Verification items for this drawing (mm, ordinates from the low corner). A direction names the side the tool comes from. Round coordinates to 2 decimals unless told otherwise and drop trailing zeros. Order: outer loops, then holes, each group sorted by start corner. A loop starts at its lowest first (then second) coordinate and runs counter-clockwise, first axis right, second up. Notation, with made-up numbers: (-20, -30) -> (6, -30) arc R8 cw to (6, -23) -> close; hole circle Ø3 at (-25.5, -0.75). An arc over 180 degrees is marked (long way). Use a Markdown table: item, result. Add a question column.
Item 1: Gauge pin test, flat ends, axial feed: pin 1 Ø3 at (x, y) = (14, 5.5) entering from -Z; pin 2 Ø3 at (x, z) = (11, 10) entering from +Y; pin 3 Ø2 at (y, z) = (3.5, 14) entering from -X. Record the tip position at first contact, or that the pin passes through.
Item 2: Sectioned sample at D-D, the plane y = 5.75. Record the cut outline in (x, z).
Item 3: Sectioned sample at C-C, the plane y = 0.5. Record the cut outline in (x, z), and give its area (3 significant figures).
Item 4: Set-up check for the marked faces 1 and 2: record each of +Z, -Z, +X, -X, +Y, -Y from which the full face is reachable in a straight line by a thin tool's end or side.
Item 5: Mould release check, pull along X, two halves, no side actions. Record for the marked faces 3, 4 and 5: pulls with the +X half, pulls with the -X half, needs draft (parallel to the pull), parting line crosses it, or undercut.
Item 6: Sectioned sample at A-A, the plane x = 10. Record the cut outline in (y, z), and give its area (3 significant figures).
Item 7: Material ranges on probe 1 along Z at (x, y) = (10, 5.1); probe 2 along Y at (x, z) = (3.5, 13.5), recorded low to high. Write a range as [from, to].
Item 8: Sectioned sample at B-B, the plane z = 10. Record the cut outline in (x, y).
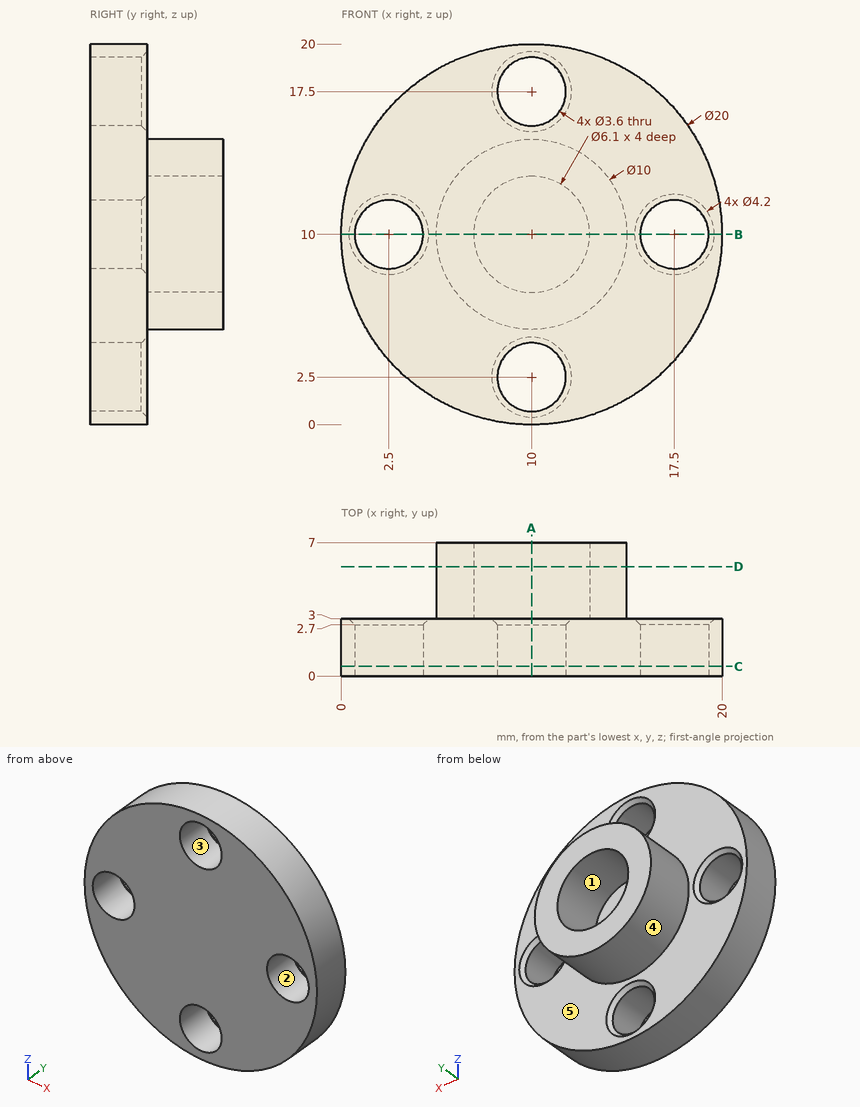
Found:
| question | item | result |
|---|---|---|
| 1 | pin 1 | stops at z = 5.67 |
| 1 | pin 2 | stops at y = 3 |
| 1 | pin 3 | stops at x = 0.5 |
| 2 | outline | circle Ø10 at (10, 10); hole circle Ø6.1 at (10, 10) |
| 3 | outline | circle Ø20 at (10, 10); hole circle Ø3.6 at (2.5, 10); hole circle Ø3.6 at (10, 2.5); hole circle Ø3.6 at (10, 17.5); hole circle Ø3.6 at (17.5, 10) |
| 3 | area | 273 mm2 |
| 4 | face 1 | +Y |
| 4 | face 2 | +Y, -Y |
| 5 | face 3 | undercut |
| 5 | face 4 | parting line crosses it |
| 5 | face 5 | needs draft |
| 6 | outline | (0, 0) -> (3, 0) -> (3, 0.4) -> (2.7, 0.7) -> (0, 0.7) -> close; (0, 4.3) -> (2.7, 4.3) -> (3, 4.6) -> (3, 5) -> (7, 5) -> (7, 6.95) -> (3, 6.95) -> (3, 13.05) -> (7, 13.05) -> (7, 15) -> (3, 15) -> (3, 15.4) -> (2.7, 15.7) -> (0, 15.7) -> close; (0, 19.3) -> (2.7, 19.3) -> (3, 19.6) -> (3, 20) -> (0, 20) -> close |
| 6 | area | 53.8 mm2 |
| 7 | probe 1 | z = [5, 6.95], [13.05, 15] |
| 7 | probe 2 | y = [0, 3] |
| 8 | outline | (0, 0) -> (0.7, 0) -> (0.7, 2.7) -> (0.4, 3) -> (0, 3) -> close; (4.3, 0) -> (15.7, 0) -> (15.7, 2.7) -> (15.4, 3) -> (15, 3) -> (15, 7) -> (13.05, 7) -> (13.05, 3) -> (6.95, 3) -> (6.95, 7) -> (5, 7) -> (5, 3) -> (4.6, 3) -> (4.3, 2.7) -> close; (19.3, 0) -> (20, 0) -> (20, 3) -> (19.6, 3) -> (19.3, 2.7) -> close |
